Verification items for the finished model (mm, model axes). A direction names the side the tool comes from. Give positions to 0.01 mm unless a question says otherwise; leave off trailing zeros. Write each loop counter-clockwise with the first axis right and the second up, starting at its lowest first coordinate (ties: lowest second). Pieces come first, ordered by that corner, then holes. Notation, with made-up numbers: (-3.75, 46.25) - (46.25, 46.25) arc R17 ccw to (46.25, 75.25) - close; hole circle Ø11 at (-35.5, -25). An arc over 180 degrees is marked (long way). Answer as a JSON object with one key per item and string values. Group by question number.
Item 1: Sectioned sample at B-B, the plane y = 0.5. Record the boundary of the cut face in (x, z).
Item 2: Draft check along Z on faces 1 (the face through (10.57, -0.46, 19.4)), 2 (the face through (10.6, -0.46, 10.57)), 3 (the face through (10.21, 18.6, 18.77)), 4 (the face through (-1, 1, 17)). Enter one of: +Z half, -Z half, draft (parallel to the pull), parting line (faces both ways), or undercut.
Item 3: Go/stop test with flat-tipped pins: pin 1 (5 mm diameter, centred on x = -2, y = 12, fed in from +Z); pin 2 (1.2 mm diameter, centred on y = 9, z = 15.5, fed in from +X); pin 3 (5.5 mm diameter, centred on x = 0, y = 10, fed in from -Z); pin 4 (2.5 mm diameter, centred on x = 6.5, z = 15.5, fed in from -Y). Record where each tip stops, or that it passes through.
Item 4: Tool access check on faces 5 (the face through (-5.113, 18.215, 15.028)), 6 (the face through (13.086, 1.495, 15.028)), 7 (the face through (4.43, -0.54, 19.4)), 8 (the face through (10, 1, 15)). Record the directions out of +Z, -Z, +X, -X, +Y, -Y that give a thin tool (end or side, any length) a straight path to the whole face; none if there is none.
Item 5: Scan lines: line 1 along Y through (x, z) = (0, 10.75); line 2 along Z through (x, y) = (13.25, -2); line 3 along Y through (x, z) = (-3, 14). Record each from-to range of solid material in increasing order. Write a range as [from, to].
Item 6: Sectioned sample at A-A, the plane z = 15. Record the boundary of the cut face in (x, y), and give its area (3 significant figures).
Item 7: Sectioned sample at C-C, the plane y = 10. Record the boundary of the cut face in (x, z), and give its area (3 significant figures).
Autodesk Inventor part; units mm, degrees
ref_plane "YZ Plane" through (0, 0, 0) normal (1, 0, 0) x (0, 1, 0)
ref_plane "XZ Plane" through (0, 0, 0) normal (0, 1, 0) x (-1, 0, 0)
ref_plane "XY Plane" through (0, 0, 0) normal (0, 0, 1) x (1, 0, 0)
ref_plane "作業平面12" through (0, 0, 10) normal (0, 0, 1) x (1, 0, 0)
sketch "スケッチ48" plane through (0, 0, 10) normal (0, 0, 1) x (1, 0, 0)
  line L0 (-10.75, -3) -> (-10.75, 15.2244)
  line L1 (-10.75, -3) -> (17.5, -3)
  line L2 (17.5, -3) -> (17.5, 11.485)
  line L3 (-10.75, 11.485) -> (-10.75, -3)
  arc A0 (17.5, 11.485) -> (0, 20.9143) centre (1.069, 1.9444) ccw
  arc A1 (0, 20.9143) -> (-10.75, 15.2244) centre (0, 7.9143) ccw
  arc A2 (17.5, 11.485) -> (0, 20.9143) centre (1.069, 1.9444) ccw
  line L4 (-10.75, 15.2244) -> (-10.75, 11.485)
  circle A3 centre (0, 10) radius 3.5
  circle A4 centre (0, 10) radius 3.5
  circle A5 centre (0, 10) radius 5.75
  point P0 (0, 0)
extrude "押し出し40" add sketch "スケッチ48" along normal blind 10 contours L0 A1 A0 L2 L1 | A5
sketch "スケッチ50" plane through (0, 0, 20) normal (0, 0, 1) x (1, 0, 0)
  line L0 (-10.75, -3) -> (17.5, -3)
  line L1 (5, -3) -> (10, -3)
  line L2 (10, -3) -> (10, 2)
  line L3 (10, 2) -> (5, 2)
  line L4 (5, 2) -> (5, -3)
  line L5 (-10.75, 15.2244) -> (-10.75, -3)
  point P0 (0, 0)
  dimension "d179" = 15.75
  dimension "d180" = 5
  dimension "d181" = 5
extrude "押し出し41" cut sketch "スケッチ50" against normal blind 10
sketch "スケッチ51" plane through (0, 0, 20) normal (0, 0, 1) x (1, 0, 0)
  circle A0 centre (0, 10) radius 5.75
  circle A1 centre (0, 10) radius 3.5
  point P0 (0, 0)
  dimension "d184" = 11.5
extrude "押し出し42" cut sketch "スケッチ51" against normal blind 7
sketch "スケッチ52" plane through (0, 0, 20) normal (0, 0, 1) x (1, 0, 0)
  line L0 (10, -3) -> (17.5, -3)
  line L1 (17.5, -3) -> (16, -3)
  line L2 (16, -3) -> (16, 11.0771)
  line L3 (16, 11.0771) -> (17.5, 11.0771)
  line L4 (17.5, 11.0771) -> (17.5, -3)
  line L5 (-10.75, -3) -> (5, -3)
  line L6 (-10.75, -3) -> (-9.25, -3)
  line L7 (-9.25, -3) -> (-9.25, 14.7471)
  line L8 (-9.25, 14.7471) -> (-10.75, 14.7471)
  line L9 (-10.75, 14.7471) -> (-10.75, -3)
  arc A0 (0, 20.9143) -> (-10.75, 15.2244) centre (0, 7.9143) ccw
  line L10 (0, 20.9143) -> (0, 19.4143)
  arc A1 (0, 19.4143) -> (-9.25, 14.7471) centre (0, 7.9143) ccw
  arc A2 (16, 11.0771) -> (0, 19.4143) centre (1.069, 1.9444) ccw
  arc A3 (17.5, 11.485) -> (0, 20.9143) centre (1.069, 1.9444) ccw
  line L11 (-10.75, 15.2244) -> (-10.75, 14.7471)
  line L12 (-10.75, 15.2244) -> (-10.75, -3)
  line L13 (17.5, -3) -> (17.5, 11.485)
  line L14 (17.5, 11.0771) -> (17.5, 11.485)
  point P0 (0, 0)
  dimension "d187" = 1.5
  dimension "d188" = 1.5
  dimension "d189" = 1.5
extrude "押し出し43" cut sketch "スケッチ52" against normal blind 7
sketch "スケッチ53" plane through (0, 0, 20) normal (0, 0, 1) x (1, 0, 0)
  line L0 (10, -3) -> (12.5, -3)
  line L1 (12.5, -3) -> (12.5, 0)
  line L2 (12.5, 0) -> (10, 0)
  line L3 (10, 0) -> (10, -3)
  line L4 (-10.75, -3) -> (5, -3)
  line L5 (5, -3) -> (0, -3)
  line L6 (0, -3) -> (0, -1)
  line L7 (0, -1) -> (5, -1)
  line L8 (5, -1) -> (5, -3)
  line L9 (12.5, -3) -> (16, -0.9793)
  line L10 (16, -3) -> (16, 11.0771)
  line L11 (10, 2) -> (10, -3)
  line L12 (10, -0.2865) -> (16, 3.1776)
  line L13 (10, -3) -> (16, -3)
  line L14 (0, -3) -> (-9.25, 2.382)
  line L15 (-9.25, 14.7471) -> (-9.25, -3)
  line L16 (5, -3) -> (5, 2)
  line L17 (5, -1.6285) -> (-9.25, 6.6628)
  point P0 (0, 0)
  dimension "d192" = 2.5
  dimension "d193" = 3
  dimension "d194" = 2
  dimension "d195" = 5
  dimension "d197" = 3.6
  dimension "d198" = 30
  dimension "d199" = 3.7
extrude "押し出し44" cut sketch "スケッチ53" against normal blind 7 contours L3 L12 L2 L1 L0 | L1 L2 L12 L10 L9 | L3 L2 L12 | L6 L7 L17 L8 L4 | L14 L15 L17 L7 L6 | L17 L7 L8
sketch "スケッチ54" plane through (0, 0, 20) normal (0, 0, 1) x (1, 0, 0)
  line L0 (-10.75, -3) -> (-10.75, 15.2244)
  line L1 (-10.75, -3) -> (-10.75, 15.2244)
  arc A0 (0, 19.4143) -> (-9.25, 14.7471) centre (0, 7.9143) ccw
  line L2 (-10.75, 15.2244) -> (-9.25, 14.7471)
  line L3 (-9.25, 14.7471) -> (-9.25, 6.6628)
  line L4 (-9.25, 14.7471) -> (-9.25, 6.6628)
  line L5 (-9.25, 6.6628) -> (3.9198, -1)
  line L6 (-9.25, 6.6628) -> (3.9198, -1)
  line L7 (3.9198, -1) -> (5, -1)
  line L8 (5, 2) -> (5, -3)
  line L9 (5, -3) -> (5, -1)
  line L10 (5, -3) -> (0, -3)
  line L11 (5, -3) -> (0, -3)
  line L12 (0, -3) -> (-9.25, 2.382)
  line L13 (-9.25, 2.382) -> (-9.25, -3)
  line L14 (-9.25, 2.382) -> (-9.25, -3)
  line L15 (-9.25, -3) -> (-10.75, -3)
  line L16 (10, -3) -> (17.5, -3)
  line L17 (17.5, 11.485) -> (17.5, -3)
  line L18 (17.5, -3) -> (17.5, 11.485)
  arc A1 (16, 11.0771) -> (0, 19.4143) centre (1.069, 1.9444) ccw
  line L19 (17.5, 11.485) -> (16, 11.0771)
  line L20 (16, 3.1776) -> (16, 11.0771)
  line L21 (16, 11.0771) -> (16, 3.1776)
  line L22 (10.4962, 0) -> (16, 3.1776)
  line L23 (16, 3.1776) -> (10.4962, 0)
  line L24 (10, 0) -> (10.4962, 0)
  line L25 (10.4962, 0) -> (10, 0)
  line L26 (10, -3) -> (10, 0)
  line L27 (10, 0) -> (10, -3)
  line L28 (12.5, -3) -> (10, -3)
  line L29 (10, -3) -> (12.5, -3)
  line L30 (16, -3) -> (16, -0.9793)
  line L31 (12.5, -3) -> (16, -0.9793)
  line L32 (16, -0.9793) -> (16, -3)
  line L33 (16, -3) -> (17.5, -3)
  arc A2 (0, 20.9143) -> (-10.75, 15.2244) centre (0, 7.9143) ccw
  arc A3 (17.5, 11.485) -> (0, 20.9143) centre (1.069, 1.9444) ccw
  arc A4 (-10.75, 0.6042) -> (-10.3133, 0) centre (0, 7.9143) ccw
  arc A5 (-9.4623, -1) -> (-9.25, -1.2201) centre (0, 7.9143) ccw
  arc A6 (10, -0.3923) -> (10.3133, 0) centre (0, 7.9143) ccw
  arc A7 (0, 19.4143) -> (-9.25, 14.7471) centre (0, 7.9143) ccw
  arc A8 (16, 11.0771) -> (0, 19.4143) centre (1.069, 1.9444) ccw
  point P0 (0, 0)
extrude "押し出し45" add sketch "スケッチ54" against normal blind 3 contours L0 L2 L3 L5 L7 L8 L10 L12 L13 L15 | A2 A3 L19 A1 A0 L2 | L17 L16 L30 L31 L26 A6 L24 L22 L20 L19 | A6 L26 L24
fillet "フィレット26" radius 2 4 edges at (5, -0.5, 20) (10, -0.5, 20) (5, -0.5, 10) (10, -0.5, 10)
fillet "フィレット27" radius 0.5 12 edges at (-10.75, 6.1122, 17) (-10.75, 6.1122, 13) (-9.25, 6.6628, 15) (-9.25, 2.382, 15) (17.5, 4.2425, 13) (17.5, 4.2425, 17) (16, 3.1776, 15) (16, -0.9793, 15) (10.0815, 18.6709, 13) (10.0815, 18.6709, 17) (-6.0815, 19.4041, 17) (-6.0815, 19.4041, 13)
properties part number "Gankenkunアンテナパーツ" material "ABS プラスチック"
Geometry check:
{
 "1": {"outline": "(-10.75, 10) - (3, 10) arc R2 ccw to (5, 12) - (5, 18) arc R2 ccw to (3, 20) - (-10.75, 20) - (-10.75, 17.5) arc R0.5 ccw to (-10.25, 17) - (-9.25, 17) - (-9.25, 13) - (-10.25, 13) arc R0.5 ccw to (-10.75, 12.5) - close; (10, 12) arc R2 ccw to (12, 10) - (17.5, 10) - (17.5, 12.5) arc R0.5 ccw to (17, 13) - (11.36, 13) - (11.36, 17) - (17, 17) arc R0.5 ccw to (17.5, 17.5) - (17.5, 20) - (12, 20) arc R2 ccw to (10, 18) - close; hole (-6.02, 13) - (1.34, 13) - (1.34, 17) - (-6.02, 17) - close"},
 "2": {"face 1": "+Z half", "face 2": "-Z half", "face 3": "draft", "face 4": "undercut"},
 "3": {"pin 1": "z = 13", "pin 2": "x = 16", "pin 3": "through", "pin 4": "y = 2"},
 "4": {"face 5": "-X, +Y", "face 6": "+X", "face 7": "+Z, -Y", "face 8": "+Z, -Z, -Y"},
 "5": {"line 1": "[-3, 6.5], [13.5, 20.91]", "line 2": "[10, 13], [17, 20]", "line 3": "[-3, -1.25], [3.03, 5.09], [14.91, 19.02]"},
 "6": {"outline": "(-9.25, -3) - (0, -3) - (-8.5, 1.94) arc R0.5 ccw to (-9.25, 1.51) - close; (-9.25, 6.95) arc R0.5 ccw to (-9, 6.52) - (3.92, -1) - (5, -1) - (5, 2) - (10, 2) - (10, 0) - (10.5, 0) - (15.75, 3.03) arc R0.5 ccw to (16, 3.47) - (16, 11.08) arc R17.5 ccw to (0, 19.41) arc R11.5 ccw to (-9.25, 14.75) - close; (12.5, -3) - (16, -3) - (16, -1.85) arc R0.5 ccw to (15.25, -1.41) - close; hole circle Ø11.5 at (0, 10)", "area": "310 mm^2"},
 "7": {"outline": "(-10.75, 10) - (-3.5, 10) - (-3.5, 13) - (-5.75, 13) - (-5.75, 20) - (-10.75, 20) - (-10.75, 17.5) arc R0.5 ccw to (-10.25, 17) - (-9.25, 17) - (-9.25, 13) - (-10.25, 13) arc R0.5 ccw to (-10.75, 12.5) - close; (3.5, 10) - (17.5, 10) - (17.5, 12.5) arc R0.5 ccw to (17, 13) - (16, 13) - (16, 17) - (17, 17) arc R0.5 ccw to (17.5, 17.5) - (17.5, 20) - (5.75, 20) - (5.75, 13) - (3.5, 13) - close", "area": "169 mm^2"}
}
